Read the model definition and answer for the solid it produces. Units are mm, in the model's axes. Face numbers are marked on the shaded views. Coordinates: 2 decimals unless noted, no trailing zeros. Order: outer loops, then holes, each group sorted by start corner. A loop starts at its lowest first (then second) coordinate and runs counter-clockwise, first axis right, second up. Notation, with made-up numbers: M 40.5,53.25 L 85.5,53.25 A25 ccw 85.5,79.25 Z; hole C -19.5,-23.5 d2. An arc over 180 degrees is marked long. One line per question, with ' | ' between items. Start each with the question number.
1) Consider probe 1 along X at (y, z) = (0.65, 18); probe 2 along Z at (x, y) = (73.5, 1.4). Determine where each line is inside the solid, lowest interval first.
2) Given P1, Ø0.5, axis at y = 0.5, z = -215.5, coming from the +X side; P2, Ø0.8, axis at x = 216, y = 0.5, coming from the -Z side, each flat-ended and moving along its own axis, determine where each tip first touches the part or whether it passes through.
3) Find section A-A, the plane z = -131.5. Write down the section's boundary in (x, y), plus the area to 3 significant figures.
4) The mould has two halves that part along Y. Classify the marked faces 1 and 2: +Y half, -Y half, draft (parallel to the pull), parting line (faces both ways), or undercut.
5) Find section B-B, the plane x = -156.5. Write down the section's boundary in (y, z), plus the area to 3 significant figures.
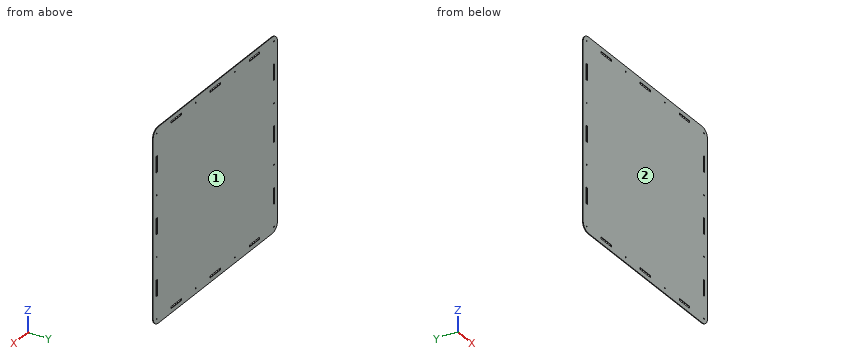
from build123d import *

# Parameters (mm, degrees)
SKETCH1_W           = 457.2
SKETCH1_H           = 457.2
BOSS_EXTRUDE1_DEPTH = 1.5875
SKETCH2_W           = 4.7625
SKETCH2_H           = 38.1
SKETCH2_W_2         = 38.1
SKETCH2_H_2         = 4.7625
CUT_EXTRUDE2_DEPTH  = 1.5875
SKETCH3_R           = 1.48828125
CUT_EXTRUDE3_DEPTH  = 1.5875
FILLET1_R           = 19.05


with BuildPart() as part:
    # Sketch1 → Boss-Extrude1 (new body)
    with BuildSketch(Plane(origin=(0, 0, 0), x_dir=(1, 0, 0), z_dir=(0, 1, 0))):
        Rectangle(SKETCH1_W, SKETCH1_H)
    extrude(amount=BOSS_EXTRUDE1_DEPTH)

    # Sketch2 → Cut-Extrude2 (cut)
    with BuildSketch(Plane(origin=(0, 1.5875, 0), x_dir=(1, 0, 0), z_dir=(0, 1, 0))):
        with Locations((-215.9, -143.933333333)):
            Rectangle(SKETCH2_W, SKETCH2_H)
        with Locations((-215.9, 0)):
            Rectangle(SKETCH2_W, SKETCH2_H)
        with Locations((-215.9, 143.933333333)):
            Rectangle(SKETCH2_W, SKETCH2_H)
        with Locations((215.9, -143.933333333)):
            Rectangle(SKETCH2_W, SKETCH2_H)
        with Locations((215.9, 0)):
            Rectangle(SKETCH2_W, SKETCH2_H)
        with Locations((215.9, 143.933333333)):
            Rectangle(SKETCH2_W, SKETCH2_H)
        with Locations((144.018, 215.9)):
            Rectangle(SKETCH2_W_2, SKETCH2_H_2)
        with Locations((0, 215.9)):
            Rectangle(SKETCH2_W_2, SKETCH2_H_2)
        with Locations((-143.891, 215.9)):
            Rectangle(SKETCH2_W_2, SKETCH2_H_2)
        with Locations((144.018, -215.9)):
            Rectangle(SKETCH2_W_2, SKETCH2_H_2)
        with Locations((-143.891, -215.9)):
            Rectangle(SKETCH2_W_2, SKETCH2_H_2)
        with Locations((0, -215.9)):
            Rectangle(SKETCH2_W_2, SKETCH2_H_2)
    extrude(amount=-CUT_EXTRUDE2_DEPTH, mode=Mode.SUBTRACT)

    # Sketch3 → Cut-Extrude3 (cut)
    with BuildSketch(Plane(origin=(0, 1.5875, 0), x_dir=(1, 0, 0), z_dir=(0, 1, 0))):
        with Locations(Location((-71.882, 215.9, 0), (0, 0, 270))):
            Circle(SKETCH3_R)
        with Locations(Location((72.136, 215.9, 0), (0, 0, 270))):
            Circle(SKETCH3_R)
        with Locations(Location((215.9, 215.9, 0), (0, 0, 270))):
            Circle(SKETCH3_R)
        with Locations(Location((215.9, 71.966666667, 0), (0, 0, 270))):
            Circle(SKETCH3_R)
        with Locations(Location((215.9, -71.966666667, 0), (0, 0, 270))):
            Circle(SKETCH3_R)
        with Locations(Location((215.9, -215.9, 0), (0, 0, 270))):
            Circle(SKETCH3_R)
        with Locations(Location((72.136, -215.9, 0), (0, 0, 270))):
            Circle(SKETCH3_R)
        with Locations(Location((-71.882, -215.9, 0), (0, 0, 270))):
            Circle(SKETCH3_R)
        with Locations(Location((-215.9, -215.9, 0), (0, 0, 270))):
            Circle(SKETCH3_R)
        with Locations(Location((-215.9, -71.966666667, 0), (0, 0, 270))):
            Circle(SKETCH3_R)
        with Locations(Location((-215.9, 71.966666667, 0), (0, 0, 270))):
            Circle(SKETCH3_R)
        with Locations(Location((-215.9, 215.9, 0), (0, 0, 270))):
            Circle(SKETCH3_R)
    extrude(amount=-CUT_EXTRUDE3_DEPTH, mode=Mode.SUBTRACT)

    # Fillet1
    fillet1_edges = [part.edges().sort_by_distance(p)[0] for p in [
        (-228.6, 0.79375, -228.6),
        (228.6, 0.79375, -228.6),
        (228.6, 0.79375, 228.6),
        (-228.6, 0.79375, 228.6),
    ]]
    fillet(fillet1_edges, radius=FILLET1_R)


solid = part.part
Report:
1) probe 1: x = -228.6 to -218.28, -213.52 to 213.52, 218.28 to 228.6 | probe 2: z = -228.6 to -216.5, -215.3 to 215.3, 216.5 to 228.6
2) P1: stops at x = 227.73 | P2: stops at z = -227.61
3) outline: M -228.6,0 L -218.28,0 L -218.28,1.59 L -228.6,1.59 Z; M -213.52,0 L 213.52,0 L 213.52,1.59 L -213.52,1.59 Z; M 218.28,0 L 228.6,0 L 228.6,1.59 L 218.28,1.59 Z | area: 711 mm^2
4) face 1: +Y half | face 2: -Y half
5) outline: M 0,-228.6 L 1.59,-228.6 L 1.59,-218.28 L 0,-218.28 Z; M 0,-213.52 L 1.59,-213.52 L 1.59,213.52 L 0,213.52 Z; M 0,218.28 L 1.59,218.28 L 1.59,228.6 L 0,228.6 Z | area: 711 mm^2
